```python
from build123d import *

# Parameters (mm, degrees)
SKETCH1_W           = 42.5
SKETCH1_H           = 35
BOSS_EXTRUDE1_DEPTH = 17.5
SKETCH3_W           = 4.2
SKETCH3_H           = 4.2
CUT_EXTRUDE1_DEPTH  = 12.5
SKETCH4_R           = 1.599999998
SKETCH4_R_2         = 1.6
CUT_EXTRUDE2_DEPTH  = 18.5
SKETCH5_R           = 2.75
CUT_EXTRUDE3_DEPTH  = 15
SKETCH6_R           = 11.25
CUT_EXTRUDE4_DEPTH  = 12
FILLET1_R           = 10


with BuildPart() as part:
    # Sketch1 → Boss-Extrude1 (new body)
    with BuildSketch(Plane.XY):
        with Locations((380.000010525, -96.878222963)):
            Rectangle(SKETCH1_W, SKETCH1_H)
    extrude(amount=BOSS_EXTRUDE1_DEPTH)

    # Sketch3 → Cut-Extrude1 (cut)
    with BuildSketch(Plane.XY.offset(17.5)):
        with Locations((397.150010525, -96.878222963)):
            Rectangle(SKETCH3_W, SKETCH3_H)
    extrude(amount=-CUT_EXTRUDE1_DEPTH, mode=Mode.SUBTRACT)

    # Sketch4 → Cut-Extrude2 (cut, through all)
    with BuildSketch(Plane.XY.offset(17.5)):
        with Locations((382.450010525, -86.878222963)):
            Circle(SKETCH4_R)
        with Locations((382.450010525, -106.878222963)):
            Circle(SKETCH4_R_2)
        with Locations((362.450010525, -86.878222963)):
            Circle(SKETCH4_R)
        with Locations((362.450010525, -106.878222963)):
            Circle(SKETCH4_R_2)
    extrude(amount=-CUT_EXTRUDE2_DEPTH, mode=Mode.SUBTRACT)

    # Sketch5 → Cut-Extrude3 (cut)
    with BuildSketch(Plane.XY.offset(17.5)):
        with Locations((382.450010525, -106.878222963)):
            Circle(SKETCH5_R)
        with Locations((382.450010525, -86.878222963)):
            Circle(SKETCH5_R)
        with Locations((362.450010525, -86.878222963)):
            Circle(SKETCH5_R)
        with Locations((362.450010525, -106.878222963)):
            Circle(SKETCH5_R)
    extrude(amount=-CUT_EXTRUDE3_DEPTH, mode=Mode.SUBTRACT)

    # Sketch6 → Cut-Extrude4 (cut)
    with BuildSketch(Plane.XY.offset(17.5)):
        with Locations((372.450010525, -96.878222963)):
            Circle(SKETCH6_R)
    extrude(amount=-CUT_EXTRUDE4_DEPTH, mode=Mode.SUBTRACT)

    # Fillet1
    fillet1_edges = [part.edges().sort_by_distance(p)[0] for p in [
        (401.250010525, -114.378222963, 8.75),
        (358.750010525, -114.378222963, 8.75),
        (358.750010525, -79.378222963, 8.75),
        (401.250010525, -79.378222963, 8.75),
    ]]
    fillet(fillet1_edges, radius=FILLET1_R)


solid = part.part
```
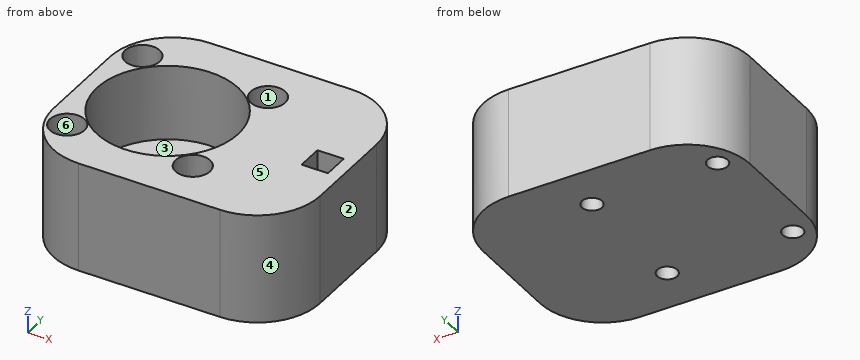
Model file for the job. Use its own axes, mm. Face numbers are marked on the shaded views. A direction names the side the tool comes from. Round coordinates to 2 decimals unless told otherwise and drop trailing zeros. Write each loop counter-clockwise with the first axis right and the second up, starting at its lowest first coordinate (ties: lowest second). Pieces come first, ordered by that corner, then holes. Notation, with made-up numbers: (-28.75, 0) -> (-13.75, 0) arc R16 cw to (-13.75, 14) -> close; hole circle Ø7 at (10.5, 60). An arc over 180 degrees is marked (long way). Answer as CSV lines item,"result".
1. Mould opens along Y. For the marked faces 3, 4, 5 and 6 say: +Y half, -Y half, draft (parallel to the pull), parting line (faces both ways), or undercut.
Resolved:
face 3,"undercut"
face 4,"-Y half"
face 5,"draft"
face 6,"undercut"
2. Drill centre lines: line 1 (X direction, y = -97.5, z = 6.5); line 2 (X direction, y = -107, z = 15); line 3 (X direction, y = -88, z = 4.25). Where is each one in solid material? Low to high.
Resolved:
line 1,"358.75 to 361.22, 383.68 to 395.05, 399.25 to 401.25"
line 2,"359.1 to 359.7, 365.2 to 367.54, 377.36 to 379.7, 385.2 to 400.9"
line 3,"358.85 to 359.94, 364.96 to 379.94, 384.96 to 401.15"
3. Slice it at D-D, the plane z = 2. List the corners of the cut face in (x, y), plus the area to 3 significant figures.
Resolved:
outline,"(358.75, -104.38) arc R10 ccw to (368.75, -114.38) -> (391.25, -114.38) arc R10 ccw to (401.25, -104.38) -> (401.25, -89.38) arc R10 ccw to (391.25, -79.38) -> (368.75, -79.38) arc R10 ccw to (358.75, -89.38) -> close; hole circle Ø3.2 at (362.45, -106.88); hole circle Ø3.2 at (362.45, -86.88); hole circle Ø3.2 at (382.45, -106.88); hole circle Ø3.2 at (382.45, -86.88)"
area,"1,370 mm²"
4. Slice it at A-A, the plane z = 16.25. List the corners of the cut face in (x, y).
Resolved:
outline,"(358.75, -104.38) arc R10 ccw to (368.75, -114.38) -> (391.25, -114.38) arc R10 ccw to (401.25, -104.38) -> (401.25, -89.38) arc R10 ccw to (391.25, -79.38) -> (368.75, -79.38) arc R10 ccw to (358.75, -89.38) -> close; hole circle Ø5.5 at (362.45, -106.88); hole circle Ø5.5 at (362.45, -86.88); hole circle Ø22.5 at (372.45, -96.88); hole circle Ø5.5 at (382.45, -106.88); hole circle Ø5.5 at (382.45, -86.88); hole (395.05, -98.98) -> (399.25, -98.98) -> (399.25, -94.78) -> (395.05, -94.78) -> close"
5. Tool access for the marked faces 1 and 2: list every direction of +Z, -Z, +X, -X, +Y, -Y with a clear straight run to the whole face (end or side of a thin tool).
Resolved:
face 1,"+Z"
face 2,"+Z, -Z, +X, +Y, -Y"
6. Slice it at B-B, the plane y = -98. List the corners of the cut face in (x, z).
Resolved:
outline,"(358.75, 0) -> (401.25, 0) -> (401.25, 17.5) -> (399.25, 17.5) -> (399.25, 5) -> (395.05, 5) -> (395.05, 17.5) -> (383.64, 17.5) -> (383.64, 5.5) -> (361.26, 5.5) -> (361.26, 17.5) -> (358.75, 17.5) -> close"
7. Pin check, flat tips, straight feed: pin 1 Ø2 at (x, z) = (396.5, 12) entering from +Y; pin 2 Ø4 at (x, y) = (382.45, -106.88) entering from +Z; pin 3 Ø3.5 at (x, z) = (398, 9.5) entering from -Y. Stop position of each tip, or through.
Resolved:
pin 1,"y = -80.33"
pin 2,"z = 2.5"
pin 3,"y = -113.04"
8. Slice it at C-C, the plane x = 397.5. List the corners of the cut face in (y, z).
Resolved:
outline,"(-112.18, 0) -> (-81.57, 0) -> (-81.57, 17.5) -> (-94.78, 17.5) -> (-94.78, 5) -> (-98.98, 5) -> (-98.98, 17.5) -> (-112.18, 17.5) -> close"
